Source: CAD feature listing. Evaluate the final solid. Frame: model axes, mm. A direction names the side the tool comes from. Give positions to 0.01 mm unless a question says otherwise; leave off trailing zeros. Order: outer loops, then holes, each group sorted by start corner. A loop starts at its lowest first (then second) coordinate and runs counter-clockwise, first axis right, second up.
```python
from build123d import *

# Parameters (mm, degrees)
SKETCH1_W               = 70
SKETCH1_H               = 56
BOSS_EXTRUDE1_DEPTH     = 5
SKETCH2_R               = 9
BOSS_EXTRUDE2_DEPTH     = 15
SKETCH4_R               = 19
CUT_EXTRUDE2_DEPTH      = 2
CUT_EXTRUDE3_DEPTH      = 49.301138703
CUT_EXTRUDE3_DEPTH_BACK = 49.301138703
SKETCH5_R               = 7.5
SKETCH6_R               = 6
CUT_EXTRUDE4_DEPTH      = 15
SKETCH7_R               = 2.5
CUT_EXTRUDE5_DEPTH      = 48.265209192


with BuildPart() as part:
    # Sketch1 → Boss-Extrude1 (new body)
    with BuildSketch(Plane(origin=(0, 0, 0), x_dir=(1, 0, 0), z_dir=(0, 1, 0))):
        Rectangle(SKETCH1_W, SKETCH1_H)
    extrude(amount=BOSS_EXTRUDE1_DEPTH)

    # Sketch2 → Boss-Extrude2 (add)
    with BuildSketch(Plane(origin=(0, 5, 0), x_dir=(1, 0, 0), z_dir=(0, 1, 0))):
        with Locations(Location((-25, -15, 0), (0, 0, 90))):
            Circle(SKETCH2_R)
    extrude(amount=BOSS_EXTRUDE2_DEPTH)

    # Sketch4 → Cut-Extrude2 (cut)
    with BuildSketch(Plane.XZ):
        with Locations(Location((0, 0, 0), (0, 0, 270))):
            Circle(SKETCH4_R)
    extrude(amount=-CUT_EXTRUDE2_DEPTH, mode=Mode.SUBTRACT)

    # Sketch5 → Cut-Extrude3 (cut, two sides: drawn at the far end of the back side and taken through both)
    with BuildSketch(Plane.XZ.offset(-2).offset(-CUT_EXTRUDE3_DEPTH_BACK)):
        with Locations(Location((0, 0, 0), (0, 0, 270))):
            Circle(SKETCH5_R)
    extrude(amount=CUT_EXTRUDE3_DEPTH + CUT_EXTRUDE3_DEPTH_BACK, mode=Mode.SUBTRACT)

    # Sketch6 → Cut-Extrude4 (cut)
    with BuildSketch(Plane(origin=(0, 20, 0), x_dir=(1, 0, 0), z_dir=(0, 1, 0))):
        with Locations(Location((-25, -15, 0), (0, 0, 270))):
            Circle(SKETCH6_R)
    extrude(amount=-CUT_EXTRUDE4_DEPTH, mode=Mode.SUBTRACT)

    # Sketch7 → Cut-Extrude5 (cut, through all)
    with BuildSketch(Plane(origin=(0, 5, 0), x_dir=(1, 0, 0), z_dir=(0, 1, 0))):
        with Locations(Location((-24, 24, 0), (0, 0, 270))):
            Circle(SKETCH7_R)
        with Locations(Location((24, 24, 0), (0, 0, 270))):
            Circle(SKETCH7_R)
        with Locations(Location((24, -24, 0), (0, 0, 270))):
            Circle(SKETCH7_R)
        with Locations(Location((-24, -24, 0), (0, 0, 270))):
            Circle(SKETCH7_R)
    extrude(amount=-CUT_EXTRUDE5_DEPTH, mode=Mode.SUBTRACT)


solid = part.part
```
1) Material intervals for L1, parallel to X at y = 2.6, z = -24; L2, parallel to X at y = 10.25, z = 15; L3, parallel to Z at x = 0, y = 3.9, sorted ascending.
Report:
L1: x = -35 to -26.5, -21.5 to 21.5, 26.5 to 35
L2: x = -34 to -31, -19 to -16
L3: z = -28 to -7.5, 7.5 to 28
2) Section query C-C, the plane x = 24. Return the cut outline in (y, z), and give its area (3 significant figures).
Report:
outline: (0, -28) - (5, -28) - (5, -26.5) - (0, -26.5) - close; (0, -21.5) - (5, -21.5) - (5, 21.5) - (0, 21.5) - close; (0, 26.5) - (5, 26.5) - (5, 28) - (0, 28) - close
area: 230 mm2
3) Section query B-B, the plane y = 3.75. Return the cut outline in (x, z), and give its area (3 significant figures).
Report:
outline: (-35, -28) - (35, -28) - (35, 28) - (-35, 28) - close; hole circle Ø5 at (-24, -24); hole circle Ø5 at (-24, 24); hole circle Ø15 at (0, 0); hole circle Ø5 at (24, -24); hole circle Ø5 at (24, 24)
area: 3,660 mm2
4) Section query D-D, the plane z = 0. Return the cut outline in (x, y).
Report:
outline: (-35, 0) - (-19, 0) - (-19, 2) - (-7.5, 2) - (-7.5, 5) - (-35, 5) - close; (7.5, 2) - (19, 2) - (19, 0) - (35, 0) - (35, 5) - (7.5, 5) - close
5) Section query A-A, the plane z = -24. Return the cut outline in (x, y).
Report:
outline: (-35, 0) - (-26.5, 0) - (-26.5, 5) - (-35, 5) - close; (-21.5, 0) - (21.5, 0) - (21.5, 5) - (-21.5, 5) - close; (26.5, 0) - (35, 0) - (35, 5) - (26.5, 5) - close
6) Pin query (flat end, axial travel): pin 1 (4.5 mm diameter, centred on x = -24, z = 24, fed in from -Y); pin 2 (1.5 mm diameter, centred on x = -3, z = 17.5, fed in from +Y); pin 3 (4.5 mm diameter, centred on x = 24, z = -24, fed in from +Y); pin 4 (1 mm diameter, centred on x = -23.5, y = 12.5, fed in from +Z). Return the tip coordinate at first contact, or that it passes through.
Report:
pin 1: stops at y = 5
pin 2: stops at y = 5
pin 3: passes through
pin 4: stops at z = 23.94
7) Reachability of faces 4 (the flat face through (-23, 20, 9)), 5 (the cylindrical face through (-27.3, 12.6, 20.54)), 6 (the cylindrical face through (-21.52, 2.54, 23.67)) from +Z, -Z, +X, -X, +Y, -Y: full face, straight path, thin tool, end or side. Return the list, or none.
Report:
face 4: +Z, -Z, +X, -X, +Y
face 5: +Y
face 6: -Y
8) Draft query along X for faces 1 (the flat face through (0, 2, 28)), 2 (the cylindrical face through (25.69, 2.54, -25.84)), 3 (the flat face through (-35, 2, 0)). Return one class per face: +X half, -X half, draft (parallel to the pull), parting line (faces both ways), or undercut.
Report:
face 1: draft
face 2: undercut
face 3: -X half
